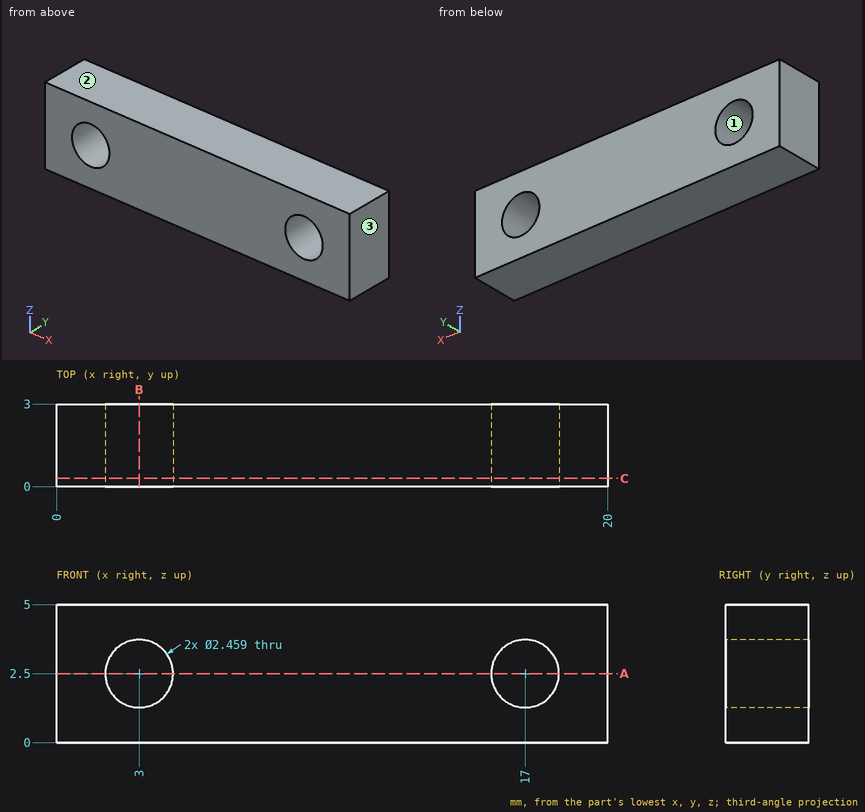
Check sheet for the drawn part. Datum: minimum x, y, z corner. Units: mm. Coordinates: 2 decimals unless noted, no trailing zeros. Order: outer loops, then holes, each group sorted by start corner. A loop starts at its lowest first (then second) coordinate and runs counter-clockwise, first axis right, second up. Notation, with made-up numbers: (87, -8.5) -> (136, -8.5) arc R19 cw to (136, -0.5) -> close; hole circle Ø2 at (-35.5, 81.25). An arc over 180 degrees is marked (long way). Use a Markdown table: item, result. Add a question column.
1. Material ranges on L1, parallel to X at y = 1.6, z = 2.5; L2, parallel to Z at x = 3, y = 1.1; L3, parallel to X at y = 1.45, z = 1.5, recorded low to high.
2. Mould release check, pull along Z, two halves, no side actions. Record for the marked faces 1, 2 and 3: pulls with the +Z half, pulls with the -Z half, needs draft (parallel to the pull), parting line crosses it, or undercut.
3. Cross-section at B-B (x = 3). Enter the section's corners in (y, z), and give its area (3 significant figures).
4. Cross-section at C-C (y = 0.3). Enter the section's corners in (x, z), and give its area (3 significant figures).
5. Cross-section at A-A (z = 2.5). Enter the section's corners in (x, y), and give its area (3 significant figures).
Filled sheet:
| question | item | result |
|---|---|---|
| 1 | L1 | 0 to 1.77, 4.23 to 15.77, 18.23 to 20 |
| 1 | L2 | 0 to 1.27, 3.73 to 5 |
| 1 | L3 | 0 to 2.28, 3.72 to 16.28, 17.72 to 20 |
| 2 | face 1 | undercut |
| 2 | face 2 | pulls with the +Z half |
| 2 | face 3 | needs draft |
| 3 | outline | (0, 0) -> (3, 0) -> (3, 1.27) -> (0, 1.27) -> close; (0, 3.73) -> (3, 3.73) -> (3, 5) -> (0, 5) -> close |
| 3 | area | 7.62 mm2 |
| 4 | outline | (0, 0) -> (20, 0) -> (20, 5) -> (0, 5) -> close; hole circle Ø2.46 at (3, 2.5); hole circle Ø2.46 at (17, 2.5) |
| 4 | area | 90.5 mm2 |
| 5 | outline | (0, 0) -> (1.77, 0) -> (1.77, 3) -> (0, 3) -> close; (4.23, 0) -> (15.77, 0) -> (15.77, 3) -> (4.23, 3) -> close; (18.23, 0) -> (20, 0) -> (20, 3) -> (18.23, 3) -> close |
| 5 | area | 45.2 mm2 |
